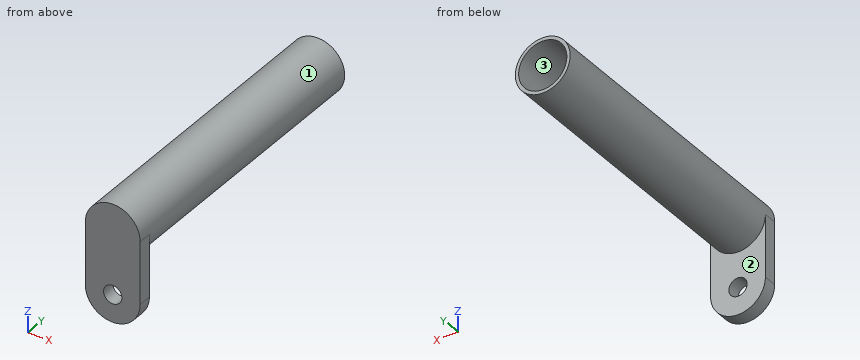
```python
from build123d import *

# Parameters (mm, degrees)
F0_R     = 4.7625
F0_R_2   = 4.188265
F1_DEPTH = 50.8
F3_DEPTH = 2.413
F4_R     = 1.5875
F5_DEPTH = 53.214


with BuildPart() as f1:
    # F0 (on Front) → F1 (new body)
    with BuildSketch(Plane.XZ):
        Circle(F0_R)
        Circle(F0_R_2, mode=Mode.SUBTRACT)
    extrude(amount=F1_DEPTH)

    # F2 (on face) → F3 (join)
    with BuildSketch(Plane.XZ.offset(50.8)):
        with BuildLine():
            Line((4.7625, -10.792703), (4.7625, 0))
            ThreePointArc((4.7625, 0), (0, 4.7625), (-4.7625, 0))
            Line((-4.7625, 0), (-4.7625, -10.792703))
            ThreePointArc((-4.7625, -10.792703), (0, -15.555203), (4.7625, -10.792703))
        make_face()
    extrude(amount=F3_DEPTH)

    # F4 (on face) → F5 (cut, through all)
    with BuildSketch(Plane.XZ.offset(53.213)):
        with Locations((0, -10.792703)):
            Circle(F4_R)
    extrude(amount=-F5_DEPTH, mode=Mode.SUBTRACT)


solid = f1.part
```
Can you work these out from the model? Positions are in its coordinate system, mm. Face numbers are marked on the shaded views. Round coordinates to 2 decimals unless told otherwise and drop trailing zeros. Loops run counter-clockwise (first coordinate to the right, second up) from the corner with the lowest first, then second, coordinate; pieces in that order, holes last. Notation, with made-up numbers: (0.5, -27) -> (14.5, -27) arc R14 ccw to (14.5, -11) -> close; hole circle Ø6 at (14.25, 55). An arc over 180 degrees is marked (long way). One line per item, written item: value. Start each with the question number.
1. If I drill on probe 1 along Z at (x, y) = (0, -33); probe 2 along Z at (x, y) = (0, -51.9); probe 3 along Y at (x, z) = (-2, -1.75), over which ranges is the centre line in solid material (lowest first)?
2. For pin 1 (1 mm diameter, centred on x = 0, z = -8.5, fed in from +Y), with a flat end and sliding along its axis, tell me the tip position at first contact or that it passes through.
3. If we section it at D-D, the plane x = 2.5: Write out the boundary of the cut face in (y, z), then the cut area to 3 significant figures.
4. If we section it at C-C, the plane z = -1.5: Write out the boundary of the cut face in (x, y).
5. If we section it at A-A, the plane x = 0: Write out the boundary of the cut face in (y, z).
6. If we mould it in two halves opening along X, with no side actions, what happens to the marked faces 1, 2 and 3? For each: pulls with the +X half, pulls with the -X half, needs draft (parallel to the pull), parting line crosses it, or undercut.
7. If we section it at B-B, the plane y = -26: Write out the boundary of the cut face in (x, z) (1 decimal), then the cut area to 3 significant figures.
Calculated:
1. probe 1: z = -4.76 to -4.19, 4.19 to 4.76
1. probe 2: z = -15.56 to -12.38, -9.21 to 4.76
1. probe 3: y = -53.21 to -50.8
2. pin 1: stops at y = -50.8
3. outline: (-53.21, -14.85) -> (-50.8, -14.85) -> (-50.8, -4.05) -> (0, -4.05) -> (0, -3.36) -> (-50.8, -3.36) -> (-50.8, 3.36) -> (0, 3.36) -> (0, 4.05) -> (-53.21, 4.05) -> close
3. area: 116 mm²
4. outline: (-4.76, -53.21) -> (4.76, -53.21) -> (4.76, -50.8) -> (4.52, -50.8) -> (4.52, 0) -> (3.91, 0) -> (3.91, -50.8) -> (-3.91, -50.8) -> (-3.91, 0) -> (-4.52, 0) -> (-4.52, -50.8) -> (-4.76, -50.8) -> close
5. outline: (-53.21, -15.56) -> (-50.8, -15.56) -> (-50.8, -12.38) -> (-53.21, -12.38) -> close; (-53.21, -9.21) -> (-50.8, -9.21) -> (-50.8, -4.76) -> (0, -4.76) -> (0, -4.19) -> (-50.8, -4.19) -> (-50.8, 4.19) -> (0, 4.19) -> (0, 4.76) -> (-53.21, 4.76) -> close
6. face 1: parting line crosses it
6. face 2: needs draft
6. face 3: undercut
7. outline: circle Ø9.5 at (0, 0); hole circle Ø8.4 at (0, 0)
7. area: 16.1 mm²
